from build123d import *

# Parameters (mm, degrees)
SKETCH1_W                        = 56
SKETCH1_H                        = 8.750000002
BOSS_EXTRUDE1_DEPTH              = 4
BOSS_EXTRUDE2_DEPTH              = 28.4
SKETCH3_W                        = 56
SKETCH3_H                        = 12
BOSS_EXTRUDE3_DEPTH              = 4
SKETCH4_W                        = 56
SKETCH4_H                        = 4
BOSS_EXTRUDE4_DEPTH              = 3.249999998
CUT_EXTRUDE1_REACH               = 38.4
SKETCH5_W                        = 4.100000004
SKETCH5_H                        = 5
CUT_EXTRUDE2_REACH               = 38.4
SKETCH6_W                        = 4.100000004
SKETCH6_H                        = 5.000000001
SKETCH7_W                        = 4.100000004
SKETCH7_H                        = 5.000000001
CUT_EXTRUDE3_DEPTH               = 37.4
SKETCH8_W                        = 4.100000004
SKETCH8_H                        = 5
CUT_EXTRUDE4_DEPTH               = 37.4
CUT_EXTRUDE5_DEPTH               = 37.4
F_2_05_2_05_DIAMETER_HOLE1_D     = 2.05
F_2_05_2_05_DIAMETER_HOLE1_DEPTH = 4
F_2_05_2_05_DIAMETER_HOLE1_TIP   = 0.615882135


with BuildPart() as part:
    # Sketch1 → Boss-Extrude1 (new body)
    with BuildSketch(Plane(origin=(0, 0, 0), x_dir=(1, 0, 0), z_dir=(0, 1, 0))):
        with Locations((0, 1.624999999)):
            Rectangle(SKETCH1_W, SKETCH1_H)
    extrude(amount=-BOSS_EXTRUDE1_DEPTH)

    # Sketch2 → Boss-Extrude2 (add)
    with BuildSketch(Plane(origin=(0, 0, 0), x_dir=(-1, 0, 0), z_dir=(0, 1, 0))):
        with BuildLine():
            Line((-17, 2.75), (17, 2.75))
            ThreePointArc((17, 2.75), (19.75, 0), (17, -2.75))
            Line((17, -2.75), (-17, -2.75))
            ThreePointArc((-17, -2.75), (-19.75, 0), (-17, 2.75))
        make_face()
    extrude(amount=BOSS_EXTRUDE2_DEPTH)

    # Sketch3 → Boss-Extrude3 (add)
    with BuildSketch(Plane.XZ.offset(-28.4)):
        Rectangle(SKETCH3_W, SKETCH3_H)
    extrude(amount=-BOSS_EXTRUDE3_DEPTH)

    # Sketch4 → Boss-Extrude4 (add)
    with BuildSketch(Plane.XY.offset(2.750000002)):
        with Locations((0, -2)):
            Rectangle(SKETCH4_W, SKETCH4_H)
    extrude(amount=BOSS_EXTRUDE4_DEPTH)

    # Sketch5 → Cut-Extrude1 (cut, up to next)
    with BuildSketch(Plane(origin=(0, 32.4, 0), x_dir=(-1, 0, 0), z_dir=(0, 1, 0)), mode=Mode.PRIVATE) as cut_extrude1_sk1:
        with Locations((25.949999998, -3.5)):
            Rectangle(SKETCH5_W, SKETCH5_H)
    cut_extrude1_tool1 = extrude(cut_extrude1_sk1.sketch, amount=-CUT_EXTRUDE1_REACH, mode=Mode.PRIVATE) & part.part
    add(cut_extrude1_tool1.solids().sort_by_distance((-25.95, 32.4, -3.5))[0], mode=Mode.SUBTRACT)

    # Sketch6 → Cut-Extrude2 (cut, up to next)
    with BuildSketch(Plane(origin=(0, 32.4, 0), x_dir=(-1, 0, 0), z_dir=(0, 1, 0)), mode=Mode.PRIVATE) as cut_extrude2_sk1:
        with Locations((-25.949999998, -3.499999999)):
            Rectangle(SKETCH6_W, SKETCH6_H)
    cut_extrude2_tool1 = extrude(cut_extrude2_sk1.sketch, amount=-CUT_EXTRUDE2_REACH, mode=Mode.PRIVATE) & part.part
    add(cut_extrude2_tool1.solids().sort_by_distance((25.95, 32.4, -3.5))[0], mode=Mode.SUBTRACT)

    # Sketch7 → Cut-Extrude3 (cut, through all)
    with BuildSketch(Plane.XZ.offset(4)):
        with Locations((25.949999998, -3.499999999)):
            Rectangle(SKETCH7_W, SKETCH7_H)
    extrude(amount=-CUT_EXTRUDE3_DEPTH, mode=Mode.SUBTRACT)

    # Sketch8 → Cut-Extrude4 (cut, through all)
    with BuildSketch(Plane.XZ.offset(4)):
        with Locations((-25.949999998, -3.5)):
            Rectangle(SKETCH8_W, SKETCH8_H)
    extrude(amount=-CUT_EXTRUDE4_DEPTH, mode=Mode.SUBTRACT)

    # Sketch9 → Cut-Extrude5 (cut, through all)
    with BuildSketch(Plane.XZ.offset(4)):
        with BuildLine():
            Line((-17, -2.000000002), (17, -2.000000002))
            ThreePointArc((17, -2.000000002), (19.000000002, 0), (17, 2.000000002))
            Line((17, 2.000000002), (-17, 2.000000002))
            ThreePointArc((-17, 2.000000002), (-19.000000002, 0), (-17, -2.000000002))
        make_face()
    extrude(amount=-CUT_EXTRUDE5_DEPTH, mode=Mode.SUBTRACT)

    # Ø2.05 (2.05) Diameter Hole1
    with Locations(Plane.XY.offset(6)):
        with Locations((26, -2), (-26, -2)):
            Hole(F_2_05_2_05_DIAMETER_HOLE1_D / 2, depth=F_2_05_2_05_DIAMETER_HOLE1_DEPTH)
            with Locations((0, 0, -(F_2_05_2_05_DIAMETER_HOLE1_DEPTH + F_2_05_2_05_DIAMETER_HOLE1_TIP / 2))):  # 118° drill point
                Cone(0, F_2_05_2_05_DIAMETER_HOLE1_D / 2, F_2_05_2_05_DIAMETER_HOLE1_TIP, mode=Mode.SUBTRACT)


solid = part.part
Source: CAD feature listing. Evaluate the final solid. Frame: model axes, mm. A direction names the side the tool comes from. Round coordinates to 2 decimals unless told otherwise and drop trailing zeros. Write each loop counter-clockwise with the first axis right and the second up, starting at its lowest first coordinate (ties: lowest second). Pieces come first, ordered by that corner, then holes. Notation, with made-up numbers: (71, -17) - (119, -17) arc R16 ccw to (119, -5) - close; hole circle Ø9 at (8.5, 70). An arc over 180 degrees is marked (long way). Use CSV: the item, a comma, the result in double quotes. Start each with the question number.
(1) Mould query, pull axis Z, two halves, no side actions, for faces 1 (the face through (27.024, -1.955, 3.972)), 2 (the face through (0, 14, -2)), 3 (the face through (0, 14, 2.75)). Classes: pulls with the +Z half, pulls with the -Z half, needs draft (parallel to the pull), parting line crosses it, or undercut.
(2) Cut plane D-D, the plane x = 22. Return loops of the section in (y, z), and give its area (3 significant figures).
(3) Material intervals for probe 1 along X at (y, z) = (-2, 4.6) (3 decimals); probe 2 along Y at (x, z) = (-26, 4.5) (3 decimals); probe 3 along Y at (x, z) = (7, 5.5), sorted ascending. Write a range as [from, to].
(4) Set-up query: faces 4 (the face through (-23.9, 30, -4)), 5 (the face through (19.75, 14, -0.06)), 6 (the face through (0, 14, 2)), 7 (the face through (26, 30, -1)). Return all of +Z, -Z, +X, -X, +Y, -Y with unobstructed straight access to the full face (end or side cutting, diameter ignored); none if empty.
(5) Cut plane A-A, the plane z = 3.75. Return loops of the section in (x, y) (3 decimals), and give its area (3 significant figures).
(6) Cut plane C-C, the plane y = 21.5. Return loops of the section in (x, z).
(7) Cut plane B-B, the plane x = 15. Return loops of the section in (y, z).
(8) First-contact query: pin 1 Ø10 at (x, y) = (-7.5, 9.5) entering from -Z; pin 2 Ø1.6 at (x, y) = (-26, -2) entering from -Z; pin 3 Ø10 at (x, y) = (3.5, 12) entering from +Z; pin 4 Ø4 at (x, z) = (-10.5, 0.5) entering from +Y. Flat tips, straight axial feed; report the tip coordinate or a pass-through.
Geometry says:
1,face 1,"needs draft"
1,face 2,"undercut"
1,face 3,"pulls with the +Z half"
2,outline,"(-4, -6) - (0, -6) - (0, 6) - (-4, 6) - close; (28.4, -6) - (32.4, -6) - (32.4, 6) - (28.4, 6) - close"
2,area,"96.0 mm²"
3,probe 1,"[-28, -27.025], [-24.975, 24.975], [27.025, 28]"
3,probe 2,"[-4, -3.025], [-0.975, 0], [28.4, 32.4]"
3,probe 3,"[-4, 0], [28.4, 32.4]"
4,face 4,"-Z, -X, +Y, -Y"
4,face 5,"+X"
4,face 6,"+Y, -Y"
4,face 7,"-Z, +X, +Y, -Y"
5,outline,"(-28, -4) - (28, -4) - (28, 0) - (-28, 0) - close; (-28, 28.4) - (28, 28.4) - (28, 32.4) - (-28, 32.4) - close; hole circle Ø2.05 at (-26, -2); hole circle Ø2.05 at (26, -2)"
5,area,"441 mm²"
6,outline,"(-17, -2.75) - (17, -2.75) arc R2.75 ccw to (17, 2.75) - (-17, 2.75) arc R2.75 ccw to start; hole (-17, -2) - (17, -2) arc R2 ccw to (17, 2) - (-17, 2) arc R2 ccw to start"
7,outline,"(-4, -6) - (0, -6) - (0, -2.75) - (28.4, -2.75) - (28.4, -6) - (32.4, -6) - (32.4, -2) - (-4, -2) - close; (-4, 2) - (32.4, 2) - (32.4, 6) - (28.4, 6) - (28.4, 2.75) - (0, 2.75) - (0, 6) - (-4, 6) - close"
8,pin 1,"z = -2.75"
8,pin 2,"z = -1"
8,pin 3,"z = 2.75"
8,pin 4,"y = 32.4"
